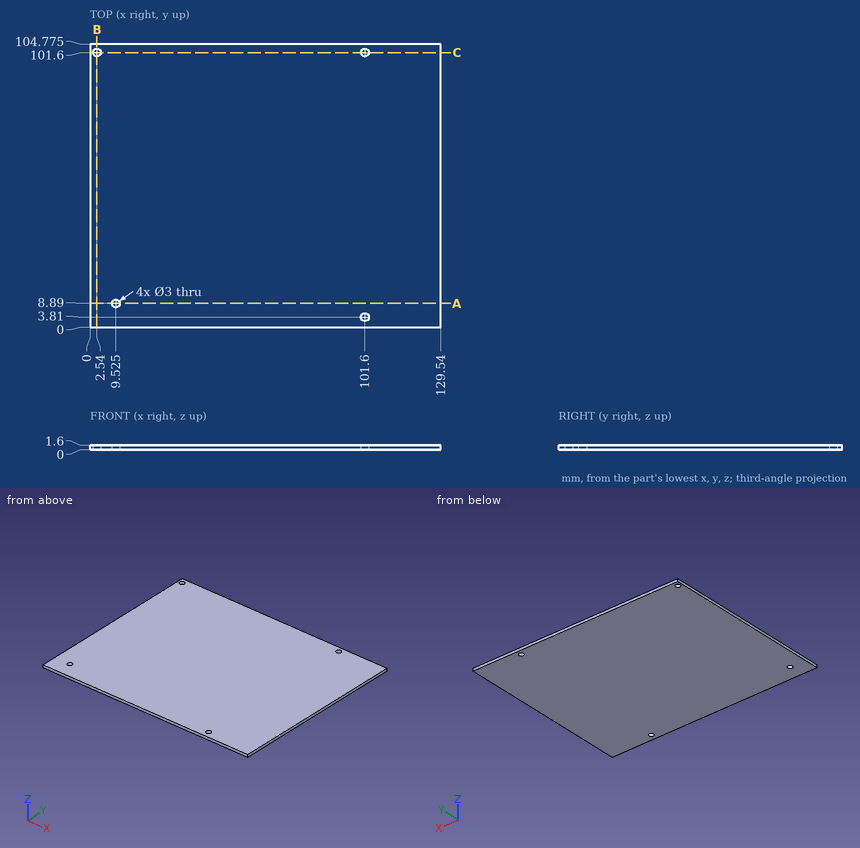
Design review of the part shown in the three views and the two pictorial views. Dimensions are in mm from the part's minimum x, y and z. Round coordinates to 2 decimals unless told otherwise and drop trailing zeros. Loops run counter-clockwise (first coordinate to the right, second up) from the corner with the lowest first, then second, coordinate; pieces in that order, holes last.
1) Wall thickness on line 1 along X through (y, z) = (101.6, 0.95); line 2 along Y through (x, z) = (101.6, 0.7) (3 decimals); line 3 along X through (y, z) = (3.81, 0.75): over which ranges is each line inside the solid? List them lowest first.
Values follow:
line 1: x = 0 to 1.04, 4.04 to 100.1, 103.1 to 129.54
line 2: y = 0 to 2.31, 5.31 to 100.1, 103.1 to 104.775
line 3: x = 0 to 100.1, 103.1 to 129.54
2) Clearance check with a flat-ended pin moving along its axis: P1, Ø1.8, axis at x = 2.54, y = 101.6, coming from the -Z side. State where the tip first meets the part, or that it passes through.
Values follow:
P1: passes through
3) Consider section C-C on y = 101.6. State the section outline as (x, z) points.
Values follow:
outline: (0, 0) - (1.04, 0) - (1.04, 1.6) - (0, 1.6) - close; (4.04, 0) - (100.1, 0) - (100.1, 1.6) - (4.04, 1.6) - close; (103.1, 0) - (129.54, 0) - (129.54, 1.6) - (103.1, 1.6) - close
4) Consider section A-A on y = 8.89. State the section outline as (x, z) points (3 decimals), then the cut area to 3 significant figures.
Values follow:
outline: (0, 0) - (8.025, 0) - (8.025, 1.6) - (0, 1.6) - close; (11.025, 0) - (129.54, 0) - (129.54, 1.6) - (11.025, 1.6) - close
area: 202 mm2
5) Consider section B-B on x = 2.54. State the section outline as (y, z) points (3 decimals).
Values follow:
outline: (0, 0) - (100.1, 0) - (100.1, 1.6) - (0, 1.6) - close; (103.1, 0) - (104.775, 0) - (104.775, 1.6) - (103.1, 1.6) - close
